Check sheet for the modelled part. Datum: model origin and axes. Units: mm. Face numbers are marked on the shaded views. Coordinates: 2 decimals unless noted, no trailing zeros. Write each loop counter-clockwise with the first axis right and the second up, starting at its lowest first coordinate (ties: lowest second). Pieces come first, ordered by that corner, then holes. Notation, with made-up numbers: M 27.25,16.5 L 75.25,16.5 A23 cw 75.25,50.5 Z; hole C 65,-24.5 d6. An arc over 180 degrees is marked long. Answer as CSV lines item,"result". Start each with the question number.
Q1. Depth check by flat-ended pin: pin 1 Ø0.6 at (x, z) = (-13.5, 664.5) entering from -Y; pin 2 Ø1 at (x, z) = (-41.5, 894.5) entering from +Y; pin 3 Ø3 at (y, z) = (49.5, 638.5) entering from +X; pin 4 Ø12 at (x, y) = (-35.5, 88) entering from +Z. Enter the tip coordinate at first touch or a pass-through.
Q2. Mould release check, pull along X, two halves, no side actions. Record for the marked faces 1 and 2: pulls with the +X half, pulls with the -X half, needs draft (parallel to the pull), parting line crosses it, or undercut.
Q3. Sectioned sample at C-C, the plane y = 183.5. Record the cut outline in (x, z).
Q4. Sectioned sample at B-B, the plane z = 284. Record the cut outline in (x, y).
Q5. Thickness scan on line 1 along Y through (x, z) = (-21.5, 680.5); line 2 along X through (y, z) = (236, 254.5); line 3 along Y through (x, z) = (-15.25, 406.5). Record the ranges inside material, lowest first. Write a range as from..to.
Q6. Sectioned sample at A-A, the plane x = -20.75. Record the cut outline in (y, z), then the cut area to 3 significant figures.
from build123d import *

# Parameters (mm, degrees)
SM_BASE_FLANGE_1_DEPTH = 896
SKETCH_4_W             = 3.1
SKETCH_4_H             = 20.2
CUT_EXTRUDE_1_DEPTH    = 10


# Sheet-metal steps are written as plain solids
with BuildPart() as part:
    # Sketch 1 → Базовая кромка1 (new body)
    with BuildSketch(Plane.XY):
        with BuildLine():
            Line((-12.578023183, 226.822978959), (-12.578023183, 248.722978959))
            ThreePointArc((-12.578023183, 248.722978959), (-13.485992161, 250.915009981), (-15.678023183, 251.822978959))
            Line((-15.678023183, 251.822978959), (-39.478023183, 251.822978959))
            ThreePointArc((-39.478023183, 251.822978959), (-41.670054205, 250.915009981), (-42.578023183, 248.722978959))
            Line((-42.578023183, 248.722978959), (-42.578023183, -45.077021041))
            ThreePointArc((-42.578023183, -45.077021041), (-41.670054205, -47.269052063), (-39.478023183, -48.177021041))
            Line((-39.478023183, -48.177021041), (-15.678023183, -48.177021041))
            ThreePointArc((-15.678023183, -48.177021041), (-13.485992161, -47.269052063), (-12.578023183, -45.077021041))
            Line((-12.578023183, -45.077021041), (-12.578023183, -23.177021041))
            Line((-12.578023183, -23.177021041), (-14.578023183, -23.177021041))
            Line((-14.578023183, -23.177021041), (-14.578023183, -45.077021041))
            ThreePointArc((-14.578023183, -45.077021041), (-14.900205724, -45.8548385), (-15.678023183, -46.177021041))
            Line((-15.678023183, -46.177021041), (-39.478023183, -46.177021041))
            ThreePointArc((-39.478023183, -46.177021041), (-40.255840642, -45.8548385), (-40.578023183, -45.077021041))
            Line((-40.578023183, -45.077021041), (-40.578023183, 248.722978959))
            ThreePointArc((-40.578023183, 248.722978959), (-40.255840642, 249.500796418), (-39.478023183, 249.822978959))
            Line((-39.478023183, 249.822978959), (-15.678023183, 249.822978959))
            ThreePointArc((-15.678023183, 249.822978959), (-14.900205724, 249.500796418), (-14.578023183, 248.722978959))
            Line((-14.578023183, 248.722978959), (-14.578023183, 226.822978959))
            Line((-14.578023183, 226.822978959), (-12.578023183, 226.822978959))
        make_face()
    extrude(amount=SM_BASE_FLANGE_1_DEPTH)

    # Эскиз4 → Вырез-Вытянуть1 (cut)
    with BuildSketch(Plane.ZY.offset(42.578023183)):
        with Locations((1.55, 201.822978959)):
            Rectangle(SKETCH_4_W, SKETCH_4_H)
        with Locations((1.55, 1.822978959)):
            Rectangle(SKETCH_4_W, SKETCH_4_H)
        with Locations((894.45, 201.822978959)):
            Rectangle(SKETCH_4_W, SKETCH_4_H)
        with Locations((894.45, 1.822978959)):
            Rectangle(SKETCH_4_W, SKETCH_4_H)
    extrude(amount=-CUT_EXTRUDE_1_DEPTH, mode=Mode.SUBTRACT)


solid = part.part
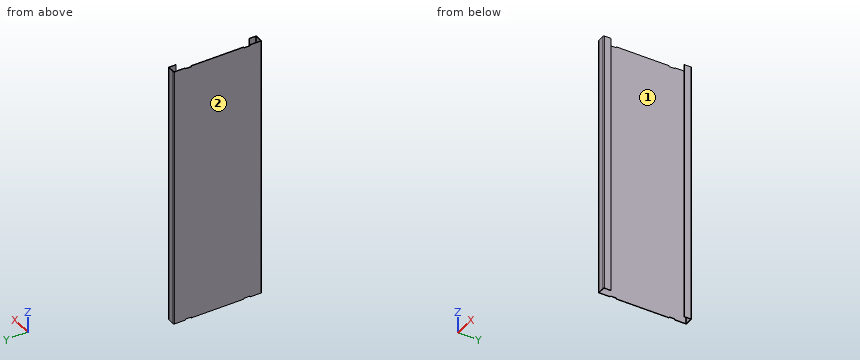
Output:
1,pin 1,"stops at y = -47.54"
1,pin 2,"stops at y = 251.42"
1,pin 3,"stops at x = -40.58"
1,pin 4,"stops at z = 896"
2,face 1,"undercut"
2,face 2,"pulls with the -X half"
3,outline,"M -42.58,0 L -40.58,0 L -40.58,896 L -42.58,896 Z"
4,outline,"M -42.58,-45.08 A3.1 ccw -39.48,-48.18 L -15.68,-48.18 A3.1 ccw -12.58,-45.08 L -12.58,-23.18 L -14.58,-23.18 L -14.58,-45.08 A1.1 cw -15.68,-46.18 L -39.48,-46.18 A1.1 cw -40.58,-45.08 L -40.58,248.72 A1.1 cw -39.48,249.82 L -15.68,249.82 A1.1 cw -14.58,248.72 L -14.58,226.82 L -12.58,226.82 L -12.58,248.72 A3.1 ccw -15.68,251.82 L -39.48,251.82 A3.1 ccw -42.58,248.72 Z"
5,line 1,"y = -48.18..-46.18, 249.82..251.82"
5,line 2,"x = -42.58..-40.58, -14.58..-12.58"
5,line 3,"y = -48.15..-46.09, 249.74..251.79"
6,outline,"M -48.18,0 L -46.18,0 L -46.18,896 L -48.18,896 Z; M 249.82,0 L 251.82,0 L 251.82,896 L 249.82,896 Z"
6,area,"3,580 mm^2"
